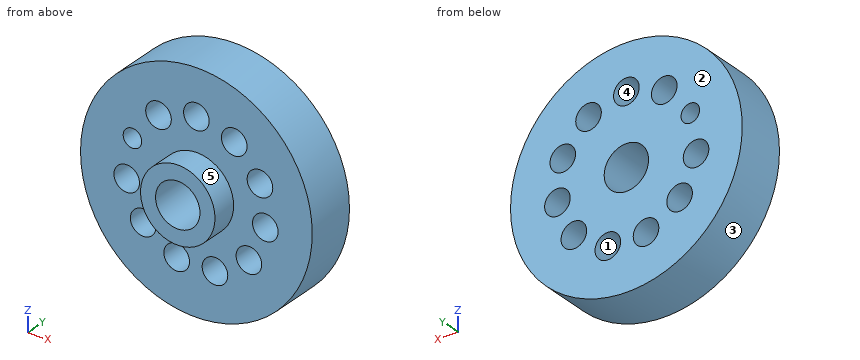
```python
from build123d import *

# Parameters (mm, degrees)
F1_R     = 57.453479
F1_R_2   = 6.35
F1_R_3   = 4.598881
F1_R_4   = 18.389548
F2_DEPTH = 25.4
F3_R     = 18.464557
F3_R_2   = 11.018284
F4_DEPTH = 38.1


with BuildPart() as f2:
    # F1 (on face) → F2 (new body)
    with BuildSketch(Plane.XZ):
        Circle(F1_R)
        with Locations((-9.742823, -32.948455)):
            Circle(F1_R_2, mode=Mode.SUBTRACT)
        with Locations((-34.542736, -4.959983)):
            Circle(F1_R_2, mode=Mode.SUBTRACT)
        with Locations((-26.394194, -22.497064)):
            Circle(F1_R_2, mode=Mode.SUBTRACT)
        with Locations((9.211395, -33.125599)):
            Circle(F1_R_2, mode=Mode.SUBTRACT)
        with Locations((26.039909, -22.497064)):
            Circle(F1_R_2, mode=Mode.SUBTRACT)
        with Locations((34.188454, -4.78284)):
            Circle(F1_R_2, mode=Mode.SUBTRACT)
        with Locations((-31.708459, 14.525663)):
            Circle(F1_R_3, mode=Mode.SUBTRACT)
        with Locations((-18.777077, 29.405612)):
            Circle(F1_R_2, mode=Mode.SUBTRACT)
        Circle(F1_R_4, mode=Mode.SUBTRACT)
        with Locations((31.531318, 14.525663)):
            Circle(F1_R_2, mode=Mode.SUBTRACT)
        with Locations((0, 34.897018)):
            Circle(F1_R_2, mode=Mode.SUBTRACT)
        with Locations((18.777075, 29.405612)):
            Circle(F1_R_2, mode=Mode.SUBTRACT)
    extrude(amount=F2_DEPTH)

    # F3 (on Front) → F4 (join)
    with BuildSketch(Plane.XZ):
        Circle(F3_R)
        Circle(F3_R_2, mode=Mode.SUBTRACT)
    extrude(amount=F4_DEPTH)


solid = f2.part
```
Read the model definition and answer for the solid it produces. Units are mm, in the model's axes. Face numbers are marked on the shaded views. A direction names the side the tool comes from. Give positions to 0.01 mm unless a question says otherwise; leave off trailing zeros. Order: outer loops, then holes, each group sorted by start corner. A loop starts at its lowest first (then second) coordinate and runs counter-clockwise, first axis right, second up.
(1) Find section D-D (x = 29.5). Give the vertices of the cut face in (y, z).
(2) For the marked faces 4 and 5, determine the directions among +Z, -Z, +X, -X, +Y, -Y from which every point of the face is accessible in a straight line to the end or side of a thin tool.
(3) Given pin 1 (1 mm diameter, centred on y = -17.5, z = 8.5, fed in from +X); pin 2 (8 mm diameter, centred on y = -10.5, z = 21, fed in from +X); pin 3 (6 mm diameter, centred on x = -20, z = 37, fed in from +Y); pin 4 (12 mm diameter, centred on x = -31.71, z = 14.53, fed in from -Y), each flat-ended and moving along its own axis, determine where each tip first touches the part or whether it passes through.
(4) Find section A-A (x = 0). Give the vertices of the cut face in (y, z), plus the area to 3 significant figures.
(5) Find section C-C (y = -34). Give the vertices of the cut face in (x, z), plus the area to 3 significant figures.
(6) Find section B-B (z = 0). Give the vertices of the cut face in (x, y).
(7) For a pull along X with two mould halves and no side action, classify the marked faces 1, 2 and 3 as released by +X, released by -X, zero draft, split by the parting line, or undercut.
(8) Straight lines are drawn through the part: L1, parallel to X at y = -18.5, z = 15; L2, parallel to X at y = -23, z = -29; L3, parallel to X at y = -7.5, z = -8. For each, find the intervals that lie inside material, in ascending order.
Result sheet:
1. outline: (-25.4, -49.3) - (0, -49.3) - (0, -27.82) - (-25.4, -27.82) - close; (-25.4, -17.17) - (0, -17.17) - (0, -9.07) - (-25.4, -9.07) - close; (-25.4, -0.5) - (0, -0.5) - (0, 8.51) - (-25.4, 8.51) - close; (-25.4, 20.54) - (0, 20.54) - (0, 49.3) - (-25.4, 49.3) - close
2. face 4: +Y, -Y
2. face 5: -Y
3. pin 1: stops at x = 56.89
3. pin 2: stops at x = 54.88
3. pin 3: stops at y = 0
3. pin 4: stops at y = -25.4
4. outline: (-38.1, -18.46) - (-25.4, -18.46) - (-25.4, -57.45) - (0, -57.45) - (0, -11.02) - (-38.1, -11.02) - close; (-38.1, 11.02) - (0, 11.02) - (0, 28.55) - (-25.4, 28.55) - (-25.4, 18.46) - (-38.1, 18.46) - close; (-25.4, 41.25) - (0, 41.25) - (0, 57.45) - (-25.4, 57.45) - close
4. area: 2,230 mm2
5. outline: circle Ø36.93 at (0, 0); hole circle Ø22.04 at (0, 0)
5. area: 690 mm2
6. outline: (-57.45, -25.4) - (-38.51, -25.4) - (-38.51, 0) - (-57.45, 0) - close; (-30.58, -25.4) - (-18.46, -25.4) - (-18.46, -38.1) - (-11.02, -38.1) - (-11.02, 0) - (-30.58, 0) - close; (11.02, -38.1) - (18.46, -38.1) - (18.46, -25.4) - (30.01, -25.4) - (30.01, 0) - (11.02, 0) - close; (38.37, -25.4) - (57.45, -25.4) - (57.45, 0) - (38.37, 0) - close
7. face 1: undercut
7. face 2: zero draft
7. face 3: split by the parting line
8. L1: x = -55.46 to -36.28, -27.13 to 25.2, 37.86 to 55.46
8. L2: x = -49.6 to -14.72, -4.77 to 4.38, 14.04 to 49.6
8. L3: x = -56.89 to -40.12, -28.97 to -7.58, 7.58 to 28.71, 39.66 to 56.89
